from build123d import *

# Parameters (mm, degrees)
SKETCH1_W           = 19.05
SKETCH1_H           = 19.05
SKETCH1_W_2         = 15.875
SKETCH1_H_2         = 15.875
BOSS_EXTRUDE1_DEPTH = 101.6
SKETCH2_R           = 3.175
CUT_EXTRUDE1_DEPTH  = 104.808420299
SKETCH3_R           = 3.175
SKETCH3_W           = 15.875
SKETCH3_H           = 9.525
CUT_EXTRUDE2_DEPTH  = 104.808420299


with BuildPart() as part:
    # Sketch1 → Boss-Extrude1 (new body)
    with BuildSketch(Plane.XY):
        Rectangle(SKETCH1_W, SKETCH1_H)
        Rectangle(SKETCH1_W_2, SKETCH1_H_2, mode=Mode.SUBTRACT)
    extrude(amount=BOSS_EXTRUDE1_DEPTH)

    # Sketch2 → Cut-Extrude1 (cut, through all)
    with BuildSketch(Plane(origin=(0, 9.525, 0), x_dir=(1, 0, 0), z_dir=(0, 1, 0))):
        with Locations(Location((0, -50.8, 0), (0, 0, 270))):
            Circle(SKETCH2_R)
    extrude(amount=-CUT_EXTRUDE1_DEPTH, mode=Mode.SUBTRACT)

    # Sketch3 → Cut-Extrude2 (cut, through all)
    with BuildSketch(Plane(origin=(9.525, 0, 0), x_dir=(0, 0, -1), z_dir=(1, 0, 0))):
        with Locations((-89.2175, 0)):
            Circle(SKETCH3_R)
        with Locations((-12.3825, 0)):
            Circle(SKETCH3_R)
        with Locations((-50.8, -4.7625)):
            Rectangle(SKETCH3_W, SKETCH3_H)
    extrude(amount=-CUT_EXTRUDE2_DEPTH, mode=Mode.SUBTRACT)


solid = part.part
CAD build for the part. Positions are in the model's coordinates, mm. A direction names the side the tool comes from. Coordinates: 2 decimals unless noted, no trailing zeros. Order: outer loops, then holes, each group sorted by start corner. A loop starts at its lowest first (then second) coordinate and runs counter-clockwise, first axis right, second up. Notation, with made-up numbers: (3.5, -13.5) -> (43.5, -13.5) arc R27 ccw to (43.5, 15.5) -> close; hole circle Ø8 at (-4.5, 14.25). An arc over 180 degrees is marked (long way). Answer in a Markdown table with one row per item.
1) Band-saw the part on D-D (z = 24). List the corners of the cut face in (x, y) (1 decimal), and give its area (3 significant figures).
Check values:
| item | result |
|---|---|
| outline | (-9.5, -9.5) -> (9.5, -9.5) -> (9.5, 9.5) -> (-9.5, 9.5) -> close; hole (-7.9, -7.9) -> (7.9, -7.9) -> (7.9, 7.9) -> (-7.9, 7.9) -> close |
| area | 111 mm2 |
2) Mould opens along Z. For faces 1 (the face through (-7.938, 2, 50)), 2 (the face through (-8.72, 0.95, 86.19)), 3 (the face through (-9, 0, 101.6)) say: pulls with the +Z half, pulls with the -Z half, needs draft (parallel to the pull), parting line crosses it, or undercut.
Check values:
| item | result |
|---|---|
| face 1 | needs draft |
| face 2 | undercut |
| face 3 | pulls with the +Z half |
3) Which spindle directions (+Z, -Z, +X, -X, +Y, -Y) get a long thin tool onto all of the face, cutting with end or side? Do faces 4 (the face through (9, 0, 51)), 5 (the face through (4, 9.525, 50)), 6 (the face through (3.4, 7.938, 50.1)). Say none if no direction does.
Check values:
| item | result |
|---|---|
| face 4 | +X, -X, -Y |
| face 5 | +Z, -Z, +X, -X, +Y |
| face 6 | +Z, -Z |
4) Band-saw the part on B-B (x = 0). List the corners of the cut face in (y, z) (1 decimal), and give its area (3 significant figures).
Check values:
| item | result |
|---|---|
| outline | (-9.5, 0) -> (-7.9, 0) -> (-7.9, 42.9) -> (-9.5, 42.9) -> close; (-9.5, 58.7) -> (-7.9, 58.7) -> (-7.9, 101.6) -> (-9.5, 101.6) -> close; (7.9, 0) -> (9.5, 0) -> (9.5, 47.6) -> (7.9, 47.6) -> close; (7.9, 54) -> (9.5, 54) -> (9.5, 101.6) -> (7.9, 101.6) -> close |
| area | 287 mm2 |
5) Band-saw the part on A-A (z = 50.8). List the corners of the cut face in (x, y) (1 decimal), and give its area (3 significant figures).
Check values:
| item | result |
|---|---|
| outline | (-9.5, 0) -> (-7.9, 0) -> (-7.9, 7.9) -> (-3.2, 7.9) -> (-3.2, 9.5) -> (-9.5, 9.5) -> close; (3.2, 7.9) -> (7.9, 7.9) -> (7.9, 0) -> (9.5, 0) -> (9.5, 9.5) -> (3.2, 9.5) -> close |
| area | 45.4 mm2 |
6) Band-saw the part on C-C (y = 6). List the corners of the cut face in (x, z) (1 decimal), and give its area (3 significant figures).
Check values:
| item | result |
|---|---|
| outline | (-9.5, 0) -> (-7.9, 0) -> (-7.9, 101.6) -> (-9.5, 101.6) -> close; (7.9, 0) -> (9.5, 0) -> (9.5, 101.6) -> (7.9, 101.6) -> close |
| area | 323 mm2 |
7) Drill centre lines: line 1 (Y direction, x = 6.5, z = 78) (1 decimal); line 2 (Z direction, x = 8.75, y = -7). Where is each one in solid material? Low to high.
Check values:
| item | result |
|---|---|
| line 1 | -9.5 to -7.9, 7.9 to 9.5 |
| line 2 | 0 to 42.86, 58.74 to 101.6 |
8) Flat gauge pins, fed straight in: P1, Ø5.5, axis at y = 0, z = 89.22, coming from the -X side; P2, Ø0.8, axis at x = 9, z = 54, coming from the -Y side; P3, Ø10, axis at x = 0, z = 50.8, coming from the -Y side. Where does each tip first touch, or does it go through?
Check values:
| item | result |
|---|---|
| P1 | through |
| P2 | y = 0 |
| P3 | y = 7.94 |
